Could you check a few things on this model? Use its own coordinates, in mm. Face numbers are marked on the shaded views. Coordinates: 2 decimals unless noted, no trailing zeros. Order: outer loops, then holes, each group sorted by start corner. A loop starts at its lowest first (then second) coordinate and runs counter-clockwise, first axis right, second up. Notation, with made-up numbers: (-17.75, -18.5) - (-2.75, -18.5) arc R9 cw to (-2.75, -3.5) - close; hole circle Ø1 at (51.25, 11.25). An arc over 180 degrees is marked (long way). Answer as a JSON object with one key per item and string values. Group by question number.
(1) Imagine slicing it at A-A, the plane z = -15. Write out the boundary of the cut face in (x, y).
(2) Please list where these lines run through material, in increasing order: probe 1 along Y at (x, z) = (4.4, -15); probe 2 along Z at (x, y) = (4.7, 92); probe 3 along Z at (x, y) = (0.6, 95.8).
(3) Imagine slicing it at B-B, the plane x = 0.95. Give the number of separate pieces and of enclosed holes in the cut face, and give its area (3 significant figures).
(4) Will these pins go through, and if not, where does the flat tip stop? P1, Ø3.5, axis at y = 6.5, z = -15, coming from the +X side; P2, Ø3, axis at x = 0.5, y = 53, coming from the +Z side; P3, Ø4, axis at y = 145, z = -20, coming from the +X side; P4, Ø2, axis at x = 5, z = -5.5, coming from the -Y side.
(5) We'd pull the mould along Z, two halves only. Please class the marked faces 1 and 2: pulls with the +Z half, pulls with the -Z half, needs draft (parallel to the pull), parting line crosses it, or undercut.
(6) Imagine slicing it at C-C, the plane y = 63.8. Write out the boundary of the cut face in (x, z).
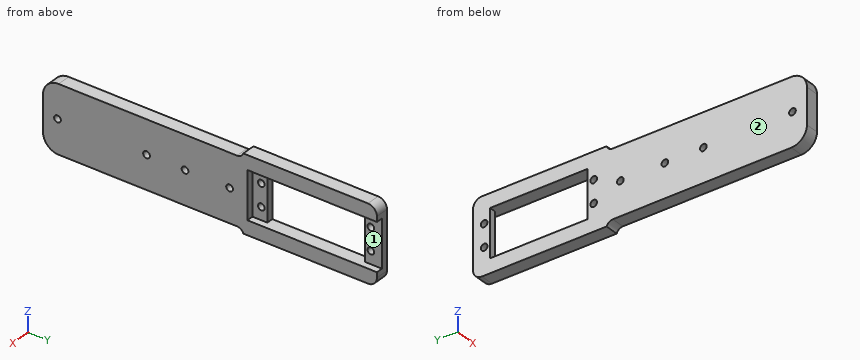
Autodesk Inventor part; units mm, degrees
ref_plane "YZ Plane" through (0, 0, 0) normal (1, 0, 0) x (0, 1, 0)
ref_plane "XZ Plane" through (0, 0, 0) normal (0, 1, 0) x (-1, 0, 0)
ref_plane "XY Plane" through (0, 0, 0) normal (0, 0, 1) x (1, 0, 0)
sketch "Sketch1" plane through (0, 0, 0) normal (1, 0, 0) x (0, 1, 0)
  line L0 (0, 0) -> (0, -30)
  line L1 (0, -30) -> (150, -30)
  line L2 (150, -30) -> (150, 0)
  line L3 (150, 0) -> (0, 0)
  dimension "d0" = 30
  dimension "d1" = 150
extrude "Extrusion1" add sketch "Sketch1" along normal blind 3
sketch "Sketch2" plane through (3, 0, 0) normal (1, 0, 0) x (0, 0, -1)
  line L0 (30, 0) -> (30, 150)
  line L1 (30, 150) -> (0, 150)
  line L2 (0, 150) -> (0, 0)
  line L3 (0, 0) -> (30, 0)
  line L4 (30, 150) -> (0, 150)
  line L5 (0, 150) -> (0, 145)
  line L6 (0, 150) -> (0, 0)
  line L7 (0, 145) -> (30, 145)
  line L8 (30, 0) -> (30, 150)
  line L9 (0, 145) -> (15, 145)
  line L10 (15, 145) -> (20, 145)
  line L11 (15, 145) -> (10, 145)
  circle A0 centre (10, 145) radius 1.5
  circle A1 centre (20, 145) radius 1.5
  circle A2 centre (20, 95.8) radius 1.5
  circle A3 centre (10, 95.8) radius 1.5
  line L12 (20, 95.8) -> (20, 97.3)
  line L13 (20, 143.5) -> (20, 145)
  line L14 (10, 95.8) -> (11.5, 95.8)
  line L15 (18.5, 95.8) -> (20, 95.8)
  line L16 (10, 145) -> (10, 143.5)
  line L17 (10, 97.3) -> (10, 95.8)
  line L18 (15, 145) -> (15, 120.4)
  line L19 (15, 120.4) -> (15, 140.9)
  line L20 (15, 140.9) -> (25.15, 140.9)
  line L21 (25.15, 140.9) -> (25.15, 99.9)
  line L22 (25.15, 99.9) -> (4.85, 99.9)
  line L23 (4.85, 99.9) -> (4.85, 140.9)
  line L24 (4.85, 140.9) -> (15, 140.9)
  dimension "d8" = 3
  dimension "d9" = 3
  dimension "d4" = 5
  dimension "d5" = 15
  dimension "d6" = 5
  dimension "d7" = 5
  dimension "d10" = 49.2
  dimension "d11" = 3
  dimension "d12" = 3
  dimension "d15" = 24.6
  dimension "d16" = 20.5
  dimension "d17" = 10.15
  dimension "d18" = 41
  dimension "d19" = 20.3
extrude "Extrusion2" cut sketch "Sketch2" against normal through all contours A1 L13 L7 | L7 A1 | L13 A1 L7 | A0 L7 | L7 L16 A0 | L7 A0 L16 | A2 L15 L12 | L12 L15 A2 | L14 L17 A3 | A3 L17 L14 | L20 L21 L22 L23 L24
sketch "Sketch3" plane through (3, 0, 0) normal (1, 0, 0) x (0, 0, -1)
  circle A0 centre (20, 145) radius 1.5
  circle A1 centre (10, 95.8) radius 1.5
  circle A2 centre (10, 145) radius 1.5
  circle A3 centre (20, 95.8) radius 1.5
  line L0 (25.15, 140.9) -> (25.15, 99.9)
  line L1 (25.15, 99.9) -> (4.85, 99.9)
  line L2 (4.85, 99.9) -> (4.85, 140.9)
  line L3 (4.85, 140.9) -> (25.15, 140.9)
  line L4 (30, 0) -> (30, 150)
  line L5 (30, 150) -> (0, 150)
  line L6 (0, 150) -> (0, 0)
  line L7 (0, 0) -> (30, 0)
  line L8 (20, 95.8) -> (15, 95.8)
  line L9 (15, 95.8) -> (15, 85.8)
  circle A4 centre (15, 85.8) radius 1.5
  line L10 (15, 85.8) -> (15, 65.8)
  circle A5 centre (15, 65.8) radius 1.5
  line L11 (20, 95.8) -> (20, 91.8)
  line L12 (20, 91.8) -> (25.15, 91.8)
  line L13 (25.15, 91.8) -> (25.15, 99.9)
  line L14 (20, 91.8) -> (4.85, 91.8)
  line L15 (25.15, 99.9) -> (4.85, 99.9)
  line L16 (4.85, 91.8) -> (4.85, 99.9)
  line L17 (25.15, 99.9) -> (25.15, 150)
  line L18 (30, 150) -> (0, 150)
  line L19 (4.85, 99.9) -> (4.85, 150)
  dimension "d22" = 5
  dimension "d23" = 10
  dimension "d24" = 3
  dimension "d34" = 20
  dimension "d35" = 3
  dimension "d41" = 4
extrude "Extrusion7" add sketch "Sketch3" along normal blind 3 contours L12 L13 L0 L17 L5 L4 L7 L6 L19 L2 L16 L14 | A4 L10 L9 | L9 L10 A4 | A5
sketch "Sketch5" plane through (0, 0, 0) normal (-1, 0, 0) x (0, 0, 1)
  circle A0 centre (-20, 145) radius 1.5
  circle A1 centre (-10, 95.8) radius 1.5
  circle A2 centre (-10, 145) radius 1.5
  circle A3 centre (-20, 95.8) radius 1.5
  line L0 (-25.15, 99.9) -> (-25.15, 140.9)
  line L1 (-25.15, 140.9) -> (-4.85, 140.9)
  line L2 (-4.85, 140.9) -> (-4.85, 99.9)
  line L3 (-4.85, 99.9) -> (-25.15, 99.9)
  line L4 (-30, 0) -> (-30, 150)
  line L5 (0, 0) -> (-30, 0)
  line L6 (0, 150) -> (0, 0)
  line L7 (-30, 150) -> (0, 150)
  line L8 (0, 146) -> (0, 0)
  line L9 (0, 0) -> (-15, 0)
  line L10 (0, 0) -> (-30, 0)
  line L11 (-15, 0) -> (-15, 6.5)
  circle A4 centre (-15, 6.5) radius 1.5
  line L12 (-15, 6.5) -> (-15, 46.5)
  circle A5 centre (-15, 46.5) radius 1.5
  dimension "d45" = 15
  dimension "d46" = 6.5
  dimension "d47" = 3
  dimension "d48" = 40
  dimension "d49" = 3
extrude "Extrusion8" cut sketch "Sketch5" against normal blind 10 contours A4 L12 L11 | L11 L12 A4 | A5
sketch "Sketch6" plane through (6, 0, 0) normal (1, 0, 0) x (0, 0, -1)
  circle A0 centre (15, 6.5) radius 1.5
  circle A1 centre (15, 46.5) radius 1.5
  line L0 (30, 150) -> (25.15, 150)
  line L1 (25.15, 150) -> (25.15, 91.8)
  line L2 (25.15, 91.8) -> (4.85, 91.8)
  line L3 (4.85, 91.8) -> (4.85, 150)
  line L4 (4.85, 150) -> (0, 150)
  line L5 (0, 150) -> (0, 0)
  line L6 (0, 0) -> (30, 0)
  line L7 (30, 0) -> (30, 150)
  line L8 (25.15, 91.8) -> (25.15, 99.9)
  line L9 (25.15, 99.9) -> (4.85, 99.9)
  line L10 (4.85, 99.9) -> (4.85, 91.8)
  line L11 (4.85, 91.8) -> (25.15, 91.8)
  circle A2 centre (10, 95.8) radius 1.5
  circle A3 centre (20, 95.8) radius 1.5
  circle A4 centre (20, 95.8) radius 1.5
  line L12 (20, 95.8) -> (15, 95.8)
  line L13 (15, 95.8) -> (15, 91.8)
  line L14 (25.15, 91.8) -> (4.85, 91.8)
  line L15 (15, 91.8) -> (15, 88.8)
  line L16 (15, 88.8) -> (15, 83.8)
  line L17 (15, 83.8) -> (15, 63.8)
  circle A5 centre (15, 63.8) radius 1.5
  circle A6 centre (15, 83.8) radius 1.5
  dimension "d52" = 5
  dimension "d53" = 3
  dimension "d54" = 5
  dimension "d55" = 20
  dimension "d56" = 3
  dimension "d57" = 3
extrude "Extrusion9" cut sketch "Sketch6" against normal blind 10 contours A6 L17 L16 | L16 L17 A6 | A5
sketch "Sketch8" plane through (6, 0, 0) normal (1, 0, 0) x (0, 0, -1)
  circle A0 centre (15, 63.8) radius 1.5
  circle A1 centre (15, 83.8) radius 1.5
  circle A2 centre (15, 6.5) radius 1.5
  circle A3 centre (15, 46.5) radius 1.5
  line L0 (30, 150) -> (25.15, 150)
  line L1 (25.15, 150) -> (25.15, 91.8)
  line L2 (25.15, 91.8) -> (4.85, 91.8)
  line L3 (4.85, 91.8) -> (4.85, 150)
  line L4 (4.85, 150) -> (0, 150)
  line L5 (0, 150) -> (0, 0)
  line L6 (0, 0) -> (30, 0)
  line L7 (30, 0) -> (30, 150)
  line L8 (4.85, 91.8) -> (25.15, 91.8)
  line L9 (25.15, 91.8) -> (25.65, 91.8)
  line L10 (25.65, 91.8) -> (25.65, 150)
  line L11 (26, 150) -> (4, 150)
  line L12 (4.85, 91.8) -> (4.35, 91.8)
  line L13 (4.35, 91.8) -> (4.35, 150)
  line L14 (4.85, 150) -> (4, 150)
  dimension "d60" = 0.5
  dimension "d61" = 0.5
extrude "Extrusion10" cut sketch "Sketch8" against normal blind 3 contours L10 L9 L1 L0 | L3 L12 L13 L4
sketch "Sketch9" plane through (3, 0, 0) normal (1, 0, 0) x (0, 0, -1)
  line L0 (4.35, 91.8) -> (25.65, 91.8)
  line L1 (25.65, 150) -> (25.65, 91.8)
  line L2 (25.65, 150) -> (4.35, 150)
  line L3 (4.35, 91.8) -> (4.35, 150)
  circle A0 centre (20, 145) radius 1.5
  circle A1 centre (10, 145) radius 1.5
  line L4 (4.85, 140.9) -> (4.85, 99.9)
  line L5 (4.85, 140.9) -> (25.15, 140.9)
  line L6 (25.15, 99.9) -> (25.15, 140.9)
  line L7 (25.15, 99.9) -> (4.85, 99.9)
  circle A2 centre (10, 95.8) radius 1.5
  circle A3 centre (20, 95.8) radius 1.5
  circle A4 centre (15, 46.5) radius 1.5
  circle A5 centre (15, 6.5) radius 1.5
  circle A6 centre (15, 83.8) radius 1.5
  circle A7 centre (15, 63.8) radius 1.5
  line L8 (25.65, 91.8) -> (4.35, 91.8)
  line L9 (4.35, 91.8) -> (4.35, 150)
  line L10 (4.35, 150) -> (0, 150)
  line L11 (0, 150) -> (0, 0)
  line L12 (0, 0) -> (30, 0)
  line L13 (30, 0) -> (30, 150)
  line L14 (30, 150) -> (25.65, 150)
  line L15 (25.65, 150) -> (25.65, 91.8)
  line L16 (4.85, 140.9) -> (25.15, 140.9)
  line L17 (4.85, 140.9) -> (4.35, 140.9)
  line L18 (25.15, 99.9) -> (25.15, 140.9)
  line L19 (25.15, 140.9) -> (25.65, 140.9)
  line L20 (25.65, 150) -> (25.65, 91.8)
  line L21 (25.15, 99.9) -> (4.85, 99.9)
  line L22 (25.15, 99.9) -> (25.65, 99.9)
  line L23 (4.85, 99.9) -> (4.35, 99.9)
extrude "Extrusion11" cut sketch "Sketch9" against normal blind 3 contours L3 L17 L4 L23 | L22 L6 L19 L1
sketch "Sketch10" plane through (3, 0, 0) normal (1, 0, 0) x (0, 0, -1)
  line L0 (4.35, 140.9) -> (25.65, 140.9)
  line L1 (25.65, 150) -> (25.65, 140.9)
  line L2 (25.65, 150) -> (4.35, 150)
  line L3 (4.35, 140.9) -> (4.35, 150)
  circle A0 centre (10, 145) radius 1.5
  circle A1 centre (20, 145) radius 1.5
  line L4 (25.65, 99.9) -> (4.35, 99.9)
  line L5 (4.35, 91.8) -> (4.35, 99.9)
  line L6 (4.35, 91.8) -> (25.65, 91.8)
  line L7 (25.65, 99.9) -> (25.65, 91.8)
  circle A2 centre (10, 95.8) radius 1.5
  circle A3 centre (20, 95.8) radius 1.5
  line L8 (4.35, 140.9) -> (4.35, 141.9)
  line L9 (4.35, 91.8) -> (4.35, 150)
  line L10 (25.65, 150) -> (25.65, 91.8)
  line L11 (25.65, 140.9) -> (25.65, 141.9)
  line L12 (4.35, 99.9) -> (4.35, 99.4)
  line L13 (4.35, 99.4) -> (25.65, 99.4)
  line L14 (25.65, 99.9) -> (25.65, 99.4)
  line L15 (4.35, 140.9) -> (4.35, 141.4)
  line L16 (4.35, 141.4) -> (25.65, 141.4)
  line L17 (25.65, 141.4) -> (25.65, 140.9)
  point P0 (0, 0)
  dimension "d67" = 0.5
  dimension "d68" = 0.5
extrude "Extrusion12" cut sketch "Sketch10" against normal blind 3 contours L3 L16 L1 L0 | L4 L7 L13 L5
sketch "Sketch11" plane through (3, 0, 0) normal (1, 0, 0) x (0, 0, -1)
  circle A0 centre (20, 145) radius 1.5
  circle A1 centre (10, 145) radius 1.5
  line L0 (4.35, 141.4) -> (25.65, 141.4)
  line L1 (25.65, 150) -> (25.65, 141.4)
  line L2 (25.65, 150) -> (4.35, 150)
  line L3 (4.35, 141.4) -> (4.35, 150)
  line L4 (25.65, 99.4) -> (4.35, 99.4)
  line L5 (4.35, 91.8) -> (4.35, 99.4)
  line L6 (4.35, 91.8) -> (25.65, 91.8)
  line L7 (25.65, 99.4) -> (25.65, 91.8)
  circle A2 centre (10, 95.8) radius 1.5
  circle A3 centre (20, 95.8) radius 1.5
  circle A4 centre (10, 95.8) radius 1.5
  line L8 (10, 97.3) -> (10, 98.5)
  line L9 (10, 98.5) -> (25.65, 98.5)
  line L10 (25.65, 150) -> (25.65, 91.8)
  line L11 (10, 98.5) -> (4.35, 98.5)
  line L12 (4.35, 91.8) -> (4.35, 150)
  circle A5 centre (10, 145) radius 1.5
  line L13 (10, 143.5) -> (10, 142.3)
  line L14 (10, 142.3) -> (25.65, 142.3)
  line L15 (10, 142.3) -> (4.35, 142.3)
  point P0 (0, 0)
  point P1 (4.35, 142.3)
  point P2 (4.35, 98.5)
  dimension "d71" = 1.2
  dimension "d72" = 1.2
extrude "Extrusion13" cut sketch "Sketch11" against normal blind 3 contours L3 L15 L14 L1 L0 | L4 L7 L9 L11 L5
sketch "Sketch12" plane through (0, 0, -30) normal (0, 0, -1) x (-1, 0, 0)
  line L0 (0, 0) -> (0, 150)
  line L1 (0, 150) -> (-6, 150)
  line L2 (-6, 0) -> (-6, 150)
  line L3 (0, 0) -> (-6, 0)
  line L4 (-6, 150) -> (-6, 90)
  line L5 (-6, 0) -> (-6, 150)
  line L6 (-6, 90) -> (0, 90)
  line L7 (0, 0) -> (0, 150)
  dimension "d75" = 60
extrude "Extrusion14" add sketch "Sketch12" along normal blind 2 contours L6 L2 L1 L0
sketch "Sketch13" plane through (0, 0, 0) normal (0, 0, 1) x (1, 0, 0)
  line L0 (0, 150) -> (0, 0)
  line L1 (0, 0) -> (6, 0)
  line L2 (6, 150) -> (6, 0)
  line L3 (0, 150) -> (6, 150)
  line L4 (6, 150) -> (6, 90)
  line L5 (6, 150) -> (6, 90)
  line L6 (6, 90) -> (0, 90)
  dimension "d78" = 60
extrude "Extrusion15" add sketch "Sketch13" along normal blind 2 contours L3 L2 L6 L0
fillet "Fillet3" radius 4 2 edges at (3, 150, 2) (3, 150, -32)
fillet "Fillet4" radius 3 2 edges at (3, 90, 0) (3, 90, -30)
fillet "Fillet5" radius 7 2 edges at (3, 0, -30) (3, 0, 0)
properties part number "antebrazo_1"
Result set:
{
 "1": {"outline": "(0, 0) - (6, 0) - (6, 5) - (0, 5) - close; (0, 8) - (6, 8) - (6, 45) - (0, 45) - close; (0, 48) - (6, 48) - (6, 62.3) - (0, 62.3) - close; (0, 65.3) - (6, 65.3) - (6, 82.3) - (0, 82.3) - close; (0, 85.3) - (6, 85.3) - (6, 91.8) - (3, 91.8) - (3, 98.5) - (0, 98.5) - close; (0, 142.3) - (3, 142.3) - (3, 150) - (0, 150) - close"},
 "2": {"probe 1": "y = 0 to 5, 8 to 45, 48 to 62.3, 65.3 to 82.3, 85.3 to 91.8", "probe 2": "z = -32 to -25.65, -4.35 to 2", "probe 3": "z = -32 to -21.5, -18.5 to -11.5, -8.5 to 2"},
 "3": {"separate pieces": "1", "enclosed holes": "9", "area": "3,730 mm^2"},
 "4": {"P1": "stops at x = 6", "P2": "stops at z = 0", "P3": "stops at x = 3", "P4": "stops at y = 0.02"},
 "5": {"face 1": "undercut", "face 2": "needs draft"},
 "6": {"outline": "(0, -30) - (6, -30) - (6, -16.5) - (0, -16.5) - close; (0, -13.5) - (6, -13.5) - (6, 0) - (0, 0) - close"}
}
